```python
from build123d import *

# Parameters (mm, degrees)
SKETCH_W               = 190
SKETCH_H               = 75
PAD_DEPTH              = 10
SKETCH001_R            = 3.3
HOLE_DEPTH             = 10.001
LINEARPATTERN_COUNT    = 2
LINEARPATTERN_PITCH    = 37
LINEARPATTERN001_COUNT = 2
LINEARPATTERN001_PITCH = 139
LINEARPATTERN002_COUNT = 2
LINEARPATTERN002_PITCH = 176
SKETCH002_R            = 3.3
HOLE001_DEPTH          = 10.001
LINEARPATTERN003_COUNT = 2
LINEARPATTERN003_PITCH = 37
LINEARPATTERN004_COUNT = 2
LINEARPATTERN004_PITCH = 139
LINEARPATTERN005_COUNT = 2
LINEARPATTERN005_PITCH = 176
SKETCH003_R            = 2.1
HOLE002_DEPTH          = 25
LINEARPATTERN006_COUNT = 2
LINEARPATTERN006_PITCH = 60


with BuildPart() as part:
    # Sketch → Pad (new body)
    with BuildSketch(Plane.XY):
        with Locations((95, 37.5)):
            Rectangle(SKETCH_W, SKETCH_H)
    extrude(amount=PAD_DEPTH)

    # Sketch001 (on Face6 of Pad) → Hole (cut, through all)
    with BuildSketch(Plane.XY.offset(10)):
        with Locations((7, 9)):
            Circle(SKETCH001_R)
    hole = extrude(amount=-HOLE_DEPTH, mode=Mode.SUBTRACT)

    # LinearPattern: Hole ×2
    with Locations(*[(i * LINEARPATTERN_PITCH, 0, 0) for i in range(1, LINEARPATTERN_COUNT)]):
        add(hole, mode=Mode.SUBTRACT)

    # LinearPattern001: Hole ×2
    with Locations(*[(i * LINEARPATTERN001_PITCH, 0, 0) for i in range(1, LINEARPATTERN001_COUNT)]):
        add(hole, mode=Mode.SUBTRACT)

    # LinearPattern002: Hole ×2
    with Locations(*[(i * LINEARPATTERN002_PITCH, 0, 0) for i in range(1, LINEARPATTERN002_COUNT)]):
        add(hole, mode=Mode.SUBTRACT)

    # Sketch002 (on Face5 of LinearPattern002) → Hole001 (cut, through all)
    with BuildSketch(Plane.XY.offset(10)):
        with Locations((7, 63)):
            Circle(SKETCH002_R)
    hole001 = extrude(amount=-HOLE001_DEPTH, mode=Mode.SUBTRACT)

    # LinearPattern003: Hole001 ×2
    with Locations(*[(i * LINEARPATTERN003_PITCH, 0, 0) for i in range(1, LINEARPATTERN003_COUNT)]):
        add(hole001, mode=Mode.SUBTRACT)

    # LinearPattern004: Hole001 ×2
    with Locations(*[(i * LINEARPATTERN004_PITCH, 0, 0) for i in range(1, LINEARPATTERN004_COUNT)]):
        add(hole001, mode=Mode.SUBTRACT)

    # LinearPattern005: Hole001 ×2
    with Locations(*[(i * LINEARPATTERN005_PITCH, 0, 0) for i in range(1, LINEARPATTERN005_COUNT)]):
        add(hole001, mode=Mode.SUBTRACT)

    # Sketch003 (on Face1 of LinearPattern005) → Hole002 (cut)
    with BuildSketch(Plane.XZ):
        with Locations((65, 5)):
            Circle(SKETCH003_R)
    hole002 = extrude(amount=-HOLE002_DEPTH, mode=Mode.SUBTRACT)

    # LinearPattern006: Hole002 ×2
    with Locations(*[(i * LINEARPATTERN006_PITCH, 0, 0) for i in range(1, LINEARPATTERN006_COUNT)]):
        add(hole002, mode=Mode.SUBTRACT)


solid = part.part
```
The listing builds one solid part. Answer for the finished solid, in the listing's coordinates (mm). A direction names the side the tool comes from. Round coordinates to 2 decimals unless told otherwise and drop trailing zeros. Loops run counter-clockwise (first coordinate to the right, second up) from the corner with the lowest first, then second, coordinate; pieces in that order, holes last. Notation, with made-up numbers: (73.25, 52.25) - (98.25, 52.25) arc R23 cw to (98.25, 67.25) - close; hole circle Ø3 at (-37.75, 85.25). An arc over 180 degrees is marked (long way). Return JSON: item names as keys, results as strings. Group by question number.
1. The part is cut by section D-D on y = 63. Determine the outline of the cut face in (x, z), then the cut area to 3 significant figures.
2. The part is cut by section C-C on z = 5. State how many separate pieces and enclosed holes the cut face has, then the cut area to 3 significant figures.
3. The part is cut by section A-A on y = 9. Determine the outline of the cut face in (x, z).
4. Each of these flat-tipped pins is pushed along its axis until it touches: P1, Ø5.5, axis at x = 44, y = 63, coming from the -Z side; P2, Ø3.5, axis at x = 65, z = 5, coming from the -Y side. Where does it stop, or does it pass through?
5. Consider probe 1 along Y at (x, z) = (7, 3); probe 2 along X at (y, z) = (19.5, 5.25); probe 3 along Y at (x, z) = (41.5, 5). Determine where each line is inside the solid, lowest interval first.
6. The part is cut by section B-B on x = 44. Determine the outline of the cut face in (y, z).
7. Which of the six approach directions +Z, -Z, +X, -X, +Y, -Y give full straight-line access (tool end or side, diameter ignored) to faces 4 (the flat face through (125, 25, 5)), 5 (the flat face through (94, 0, 5))?
8. The mould has two halves that part along Z. Classify faces 1 (the flat face through (65, 25, 5)), 2 (the cylindrical face through (143.57, 11.23, 5.07)), 3 (the flat face through (94, 38, 0)): pulls with the +Z half, pulls with the -Z half, needs draft (parallel to the pull), parting line crosses it, or undercut.
Resolved:
{
 "1": {"outline": "(0, 0) - (3.7, 0) - (3.7, 10) - (0, 10) - close; (10.3, 0) - (40.7, 0) - (40.7, 10) - (10.3, 10) - close; (47.3, 0) - (142.7, 0) - (142.7, 10) - (47.3, 10) - close; (149.3, 0) - (179.7, 0) - (179.7, 10) - (149.3, 10) - close; (186.3, 0) - (190, 0) - (190, 10) - (186.3, 10) - close", "area": "1,640 mm²"},
 "2": {"separate pieces": "1", "enclosed holes": "8", "area": "13,800 mm²"},
 "3": {"outline": "(0, 0) - (3.7, 0) - (3.7, 10) - (0, 10) - close; (10.3, 0) - (40.7, 0) - (40.7, 10) - (10.3, 10) - close; (47.3, 0) - (142.7, 0) - (142.7, 10) - (47.3, 10) - close; (149.3, 0) - (179.7, 0) - (179.7, 10) - (149.3, 10) - close; (186.3, 0) - (190, 0) - (190, 10) - (186.3, 10) - close; hole circle Ø4.2 at (65, 5); hole circle Ø4.2 at (125, 5)"},
 "4": {"P1": "passes through", "P2": "stops at y = 25"},
 "5": {"probe 1": "y = 0 to 5.7, 12.3 to 59.7, 66.3 to 75", "probe 2": "x = 0 to 62.91, 67.09 to 122.91, 127.09 to 190", "probe 3": "y = 0 to 6.85, 11.15 to 60.85, 65.15 to 75"},
 "6": {"outline": "(0, 0) - (5.7, 0) - (5.7, 10) - (0, 10) - close; (12.3, 0) - (59.7, 0) - (59.7, 10) - (12.3, 10) - close; (66.3, 0) - (75, 0) - (75, 10) - (66.3, 10) - close"},
 "7": {"face 4": "-Y", "face 5": "+Z, -Z, +X, -X, -Y"},
 "8": {"face 1": "undercut", "face 2": "needs draft", "face 3": "pulls with the -Z half"}
}
